Read the model definition and answer for the solid it produces. Units are mm, in the model's axes. A direction names the side the tool comes from. Give positions to 0.01 mm unless a question says otherwise; leave off trailing zeros. Loops run counter-clockwise (first coordinate to the right, second up) from the corner with the lowest first, then second, coordinate; pieces in that order, holes last.
(1) Each of these flat-tipped pins is pushed along its axis until it touches: P1, Ø3, axis at y = -9, z = 4.5, coming from the +X side; P2, Ø5, axis at x = -29.72, z = 5, coming from the +Y side. Where does it stop, or does it pass through?
(2) Straight lines are drawn through the part: probe 1 along X at (y, z) = (-2.55, 5); probe 2 along Y at (x, z) = (-51.95, 5); probe 3 along Y at (x, z) = (-39, 7.75). For each, find the intervals that lie inside material, in ascending order.
(3) Determine the mould class of faces 3 (the face through (-24.736, -3, 5)), 4 (the face through (-27.74, -3.03, 4.74)), 5 (the face through (-43, -4, 10)), 6 (the face through (-43, -4, 0)) for opening direction Z: pulls with the +Z half, pulls with the -Z half, needs draft (parallel to the pull), parting line crosses it, or undercut.
(4) Find section A-A, the plane z = 5. Write down the section's boundary in (x, y).
(5) Find section D-D, the plane z = 8.5. Write down the section's boundary in (x, y), then the cut area to 3 significant figures.
(6) Find section C-C, the plane x = -38.5. Write down the section's boundary in (y, z), then the cut area to 3 significant figures.
(7) Which of the six approach directions +Z, -Z, +X, -X, +Y, -Y give full straight-line access (tool end or side, diameter ignored) to faces 1 (the face through (-52.25, -12.32, 5.69)), 2 (the face through (-37, -5.986, 5))?
(8) Find section B-B, the plane y = -10.25. Write down the section's boundary in (x, z), then the cut area to 3 significant figures.
```python
from build123d import *

# Parameters (mm, degrees)
BOSS_EXTRUDE1_DEPTH     = 10
CUT_EXTRUDE1_DEPTH      = 58.959168463
CUT_EXTRUDE1_DEPTH_BACK = 58.959168463
SKETCH7_R               = 0.991796169
CUT_EXTRUDE2_DEPTH      = 58.959168463
CUT_EXTRUDE2_DEPTH_BACK = 58.959168463
CUT_EXTRUDE3_DEPTH      = 36.542676149
CUT_EXTRUDE3_DEPTH_BACK = 36.542676149
SKETCH9_R               = 0.986488891
CUT_EXTRUDE4_DEPTH      = 36.542676149
CUT_EXTRUDE4_DEPTH_BACK = 36.542676149
SKETCH10_R              = 1.5
CUT_EXTRUDE5_DEPTH      = 58.959168463
CUT_EXTRUDE5_DEPTH_BACK = 58.959168463
SKETCH12_R              = 2


with BuildPart() as part:
    # Sketch1 → Boss-Extrude1 (new body)
    with BuildSketch(Plane.XY):
        Polygon((-54.735576923, 0), (-24.735576923, 0), (-24.735576923, -5.985576923), (-49.831730769, -5.985576923), (-49.831730769, -16.225961538), (-54.735576923, -16.225961538), align=None)
    extrude(amount=BOSS_EXTRUDE1_DEPTH)

    # Sketch7 → Cut-Extrude1 (cut, two sides: drawn at the far end of the back side and taken through both)
    with BuildSketch(Plane(origin=(0, 0, 0), x_dir=(1, 0, 0), z_dir=(0, 1, 0)).offset(-CUT_EXTRUDE1_DEPTH_BACK)):
        with Locations(Location((-29.721531387, -5, 0), (0, 0, 270))):
            Circle(SKETCH7_R)
    extrude(amount=CUT_EXTRUDE1_DEPTH + CUT_EXTRUDE1_DEPTH_BACK, mode=Mode.SUBTRACT)

    # Sketch2 → Cut-Extrude2 (cut, two sides: drawn at the far end of the back side and taken through both)
    with BuildSketch(Plane(origin=(0, 0, 0), x_dir=(1, 0, 0), z_dir=(0, 1, 0)).offset(-CUT_EXTRUDE2_DEPTH_BACK)):
        with BuildLine():
            ThreePointArc((-45.014660465, -5), (-46.003925048, -4.010735417), (-46.993189631, -5))
            Line((-46.993189631, -5), (-45.014660465, -5))
        make_face()
        with BuildLine():
            Line((-45.014660465, -5), (-46.993189631, -5))
            ThreePointArc((-46.993189631, -5), (-46.003925048, -5.989264583), (-45.014660465, -5))
        make_face()
    extrude(amount=CUT_EXTRUDE2_DEPTH + CUT_EXTRUDE2_DEPTH_BACK, mode=Mode.SUBTRACT)

    # Sketch9 → Cut-Extrude3 (cut, two sides: drawn at the far end of the back side and taken through both)
    with BuildSketch(Plane.ZY.offset(54.735576923).offset(-CUT_EXTRUDE3_DEPTH_BACK)):
        with Locations((5, -10.990115231)):
            Circle(SKETCH9_R)
    extrude(amount=CUT_EXTRUDE3_DEPTH + CUT_EXTRUDE3_DEPTH_BACK, mode=Mode.SUBTRACT)

    # Sketch10 → Cut-Extrude4 (cut, two sides: drawn at the far end of the back side and taken through both)
    with BuildSketch(Plane.ZY.offset(54.735576923).offset(-CUT_EXTRUDE4_DEPTH_BACK)):
        with Locations((5, -10.990115231)):
            Circle(SKETCH10_R)
    extrude(amount=CUT_EXTRUDE4_DEPTH + CUT_EXTRUDE4_DEPTH_BACK, mode=Mode.SUBTRACT)

    # Sketch12 → Cut-Extrude5 (cut, two sides: drawn at the far end of the back side and taken through both)
    with BuildSketch(Plane(origin=(0, 0, 0), x_dir=(1, 0, 0), z_dir=(0, 1, 0)).offset(-CUT_EXTRUDE5_DEPTH_BACK)):
        with Locations(Location((-46.003925048, -5, 0), (0, 0, 270))):
            Circle(SKETCH12_R)
        with Locations(Location((-29.721531387, -5, 0), (0, 0, 270))):
            Circle(SKETCH12_R)
    extrude(amount=CUT_EXTRUDE5_DEPTH + CUT_EXTRUDE5_DEPTH_BACK, mode=Mode.SUBTRACT)


solid = part.part
```
Entries:
1. P1: stops at x = -49.83
1. P2: stops at y = 0
2. probe 1: x = -54.74 to -48, -44 to -31.72, -27.72 to -24.74
2. probe 2: y = -16.23 to -12.49, -9.49 to 0
2. probe 3: y = -5.99 to 0
3. face 3: needs draft
3. face 4: undercut
3. face 5: pulls with the +Z half
3. face 6: pulls with the -Z half
4. outline: (-54.74, -16.23) - (-49.83, -16.23) - (-49.83, -12.49) - (-54.74, -12.49) - close; (-54.74, -9.49) - (-49.83, -9.49) - (-49.83, -5.99) - (-48, -5.99) - (-48, 0) - (-54.74, 0) - close; (-44, -5.99) - (-31.72, -5.99) - (-31.72, 0) - (-44, 0) - close; (-27.72, -5.99) - (-24.74, -5.99) - (-24.74, 0) - (-27.72, 0) - close
5. outline: (-54.74, -16.23) - (-49.83, -16.23) - (-49.83, -5.99) - (-24.74, -5.99) - (-24.74, 0) - (-54.74, 0) - close
5. area: 230 mm2
6. outline: (-5.99, 0) - (0, 0) - (0, 10) - (-5.99, 10) - close
6. area: 59.9 mm2
7. face 1: +X, -X
7. face 2: +Z, -Z, +X, -Y
8. outline: (-54.74, 0) - (-49.83, 0) - (-49.83, 3.7) - (-54.74, 3.7) - close; (-54.74, 6.3) - (-49.83, 6.3) - (-49.83, 10) - (-54.74, 10) - close
8. area: 36.2 mm2
